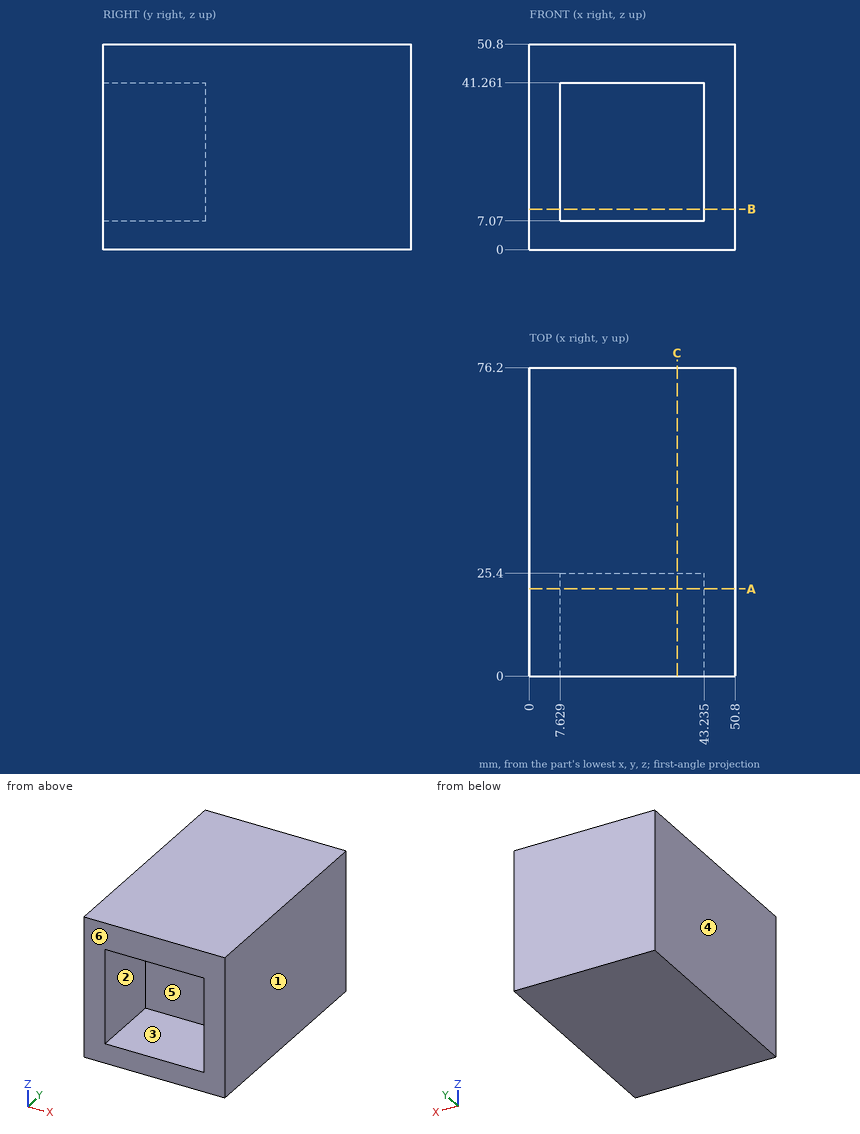
Job drawing, mm, ordinate dimensions from the low corner. One solid piece. A direction names the side the tool comes from. Give positions to 0.01 mm unless a question says otherwise; leave off trailing zeros. Order: outer loops, then holes, each group sorted by start corner. A loop starts at its lowest first (then second) coordinate and runs counter-clockwise, first axis right, second up. Notation, with made-up numbers: (74, -18.5) - (103, -18.5) arc R23 cw to (103, 12.5) - close; hole circle Ø10 at (-38, 88.25). An arc over 180 degrees is marked (long way). One line per question, with ' | ' between items.
1. Drop flat-ended pins along their axis: P1, Ø12.5, axis at y = 12, z = 21.5, coming from the -X side; P2, Ø1.5, axis at x = 23.5, z = 30.5, coming from the -Y side. Give the stop position or say it passes through.
Filled in:
P1: x = 0 | P2: y = 25.4
2. Band-saw the part on C-C on x = 36.5. List the corners of the cut face in (y, z).
Filled in:
outline: (0, 0) - (76.2, 0) - (76.2, 50.8) - (0, 50.8) - (0, 41.26) - (25.4, 41.26) - (25.4, 7.07) - (0, 7.07) - close
3. Which spindle directions (+Z, -Z, +X, -X, +Y, -Y) get a long thin tool onto all of the face, cutting with end or side? Do the marked faces 1 and 2. Say none if no direction does.
Filled in:
face 1: +Z, -Z, +X, +Y, -Y | face 2: -Y
4. Pull direction X, two halves, no side cores. Call the marked faces 3, 4, 5 and 6: +X half, -X half, draft (parallel to the pull), parting line (faces both ways), or undercut.
Filled in:
face 3: undercut | face 4: -X half | face 5: undercut | face 6: draft
5. Drill centre lines: probe 1 along Z at (x, y) = (22, 23.5); probe 2 along X at (y, z) = (12, 38.5) (1 decimal); probe 3 along Y at (x, z) = (24, 27.5). Where is each one in solid material? Low to high.
Filled in:
probe 1: 0 to 7.07, 41.26 to 50.8 | probe 2: 0 to 7.6, 43.2 to 50.8 | probe 3: 25.4 to 76.2
6. Band-saw the part on A-A on y = 21.5. List the corners of the cut face in (x, z) (1 decimal).
Filled in:
outline: (0, 0) - (50.8, 0) - (50.8, 50.8) - (0, 50.8) - close; hole (7.6, 7.1) - (43.2, 7.1) - (43.2, 41.3) - (7.6, 41.3) - close
7. Band-saw the part on B-B on z = 10. List the corners of the cut face in (x, y) (1 decimal).
Filled in:
outline: (0, 0) - (7.6, 0) - (7.6, 25.4) - (43.2, 25.4) - (43.2, 0) - (50.8, 0) - (50.8, 76.2) - (0, 76.2) - close
